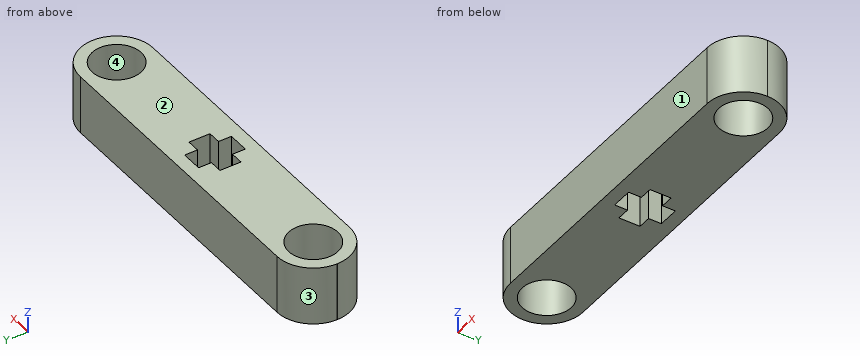
from build123d import *

# Parameters (mm, degrees)
F0_R     = 2.667
F1_DEPTH = 6.35


with BuildPart() as f1:
    # F0 (on Top) → F1 (new body)
    with BuildSketch(Plane.XY):
        with BuildLine():
            Line((-16.1417, -3.937), (16.129, -3.937))
            ThreePointArc((16.129, -3.937), (18.912879, -2.783879), (20.066, 0))
            ThreePointArc((20.066, 0), (18.912879, 2.783879), (16.129, 3.937))
            Line((16.129, 3.937), (-16.1417, 3.937))
            ThreePointArc((-16.1417, 3.937), (-18.916599, 2.787599), (-20.066, 0.0127))
            Line((-20.066, 0.0127), (-20.066, -0.0127))
            ThreePointArc((-20.066, -0.0127), (-18.916599, -2.787599), (-16.1417, -3.937))
        make_face()
        with Locations((-16.129, 0)):
            Circle(F0_R, mode=Mode.SUBTRACT)
        Polygon((-1.143, 2.54), (0, 2.54), (1.143, 2.54), (1.143, 1.143), (2.54, 1.143), (2.54, 0), (2.54, -1.143), (1.143, -1.143), (1.143, -2.54), (0, -2.54), (-1.143, -2.54), (-1.143, -1.143), (-2.54, -1.143), (-2.54, 0), (-2.54, 1.143), (-1.143, 1.143), align=None, mode=Mode.SUBTRACT)
        with Locations((16.129, 0)):
            Circle(F0_R, mode=Mode.SUBTRACT)
    extrude(amount=F1_DEPTH)


solid = f1.part
Verification items for the finished model (mm, model axes). Face numbers are marked on the shaded views. Give positions to 0.01 mm unless a question says otherwise; leave off trailing zeros. Loops run counter-clockwise (first coordinate to the right, second up) from the corner with the lowest first, then second, coordinate; pieces in that order, holes last.
1) Sectioned sample at C-C, the plane y = 3.25. Enter the section's corners in (x, z), then the cut area to 3 significant figures.
2) Draft check along Y on the marked faces 1, 2, 3 and 4. Enter one of: pulls with the +Y half, pulls with the -Y half, needs draft (parallel to the pull), parting line crosses it, or undercut.
3) Thickness scan on line 1 along Y through (x, z) = (1.5, 4.5); line 2 along X through (y, z) = (1.75, 0.5); line 3 along Y through (x, z) = (0.5, 3.5). Record the ranges inside material, lowest first.
4) Sectioned sample at B-B, the plane y = -2. Enter the section's corners in (x, z).
5) Sectioned sample at A-A, the plane z = 4. Count the separate pieces of the cut face and the enclosed holes in it, then the cut area to 3 significant figures.
6) Depth check by flat-ended pin: pin 1 Ø2 at (y, z) = (1, 4.5) entering from -X; pin 2 Ø0.7 at (y, z) = (-0.5, 3.5) entering from +X; pin 3 Ø0.7 at (y, z) = (-1.5, 2.5) entering from +X; pin 4 Ø0.7 at (y, z) = (2, 2) entering from +X. Enter the tip coordinate at first touch or a pass-through.
Answers:
1. outline: (-18.36, 0) - (18.35, 0) - (18.35, 6.35) - (-18.36, 6.35) - close
1. area: 233 mm2
2. face 1: pulls with the -Y half
2. face 2: needs draft
2. face 3: pulls with the +Y half
2. face 4: undercut
3. line 1: y = -3.94 to -1.14, 1.14 to 3.94
3. line 2: x = -19.66 to -18.14, -14.12 to -1.14, 1.14 to 14.12, 18.14 to 19.66
3. line 3: y = -3.94 to -2.54, 2.54 to 3.94
4. outline: (-19.53, 0) - (-17.89, 0) - (-17.89, 6.35) - (-19.53, 6.35) - close; (-14.36, 0) - (-1.14, 0) - (-1.14, 6.35) - (-14.36, 6.35) - close; (1.14, 0) - (14.36, 0) - (14.36, 6.35) - (1.14, 6.35) - close; (17.89, 0) - (19.52, 0) - (19.52, 6.35) - (17.89, 6.35) - close
5. separate pieces: 1
5. enclosed holes: 3
5. area: 240 mm2
6. pin 1: stops at x = -20.07
6. pin 2: stops at x = 20.06
6. pin 3: stops at x = 19.89
6. pin 4: stops at x = 19.7
